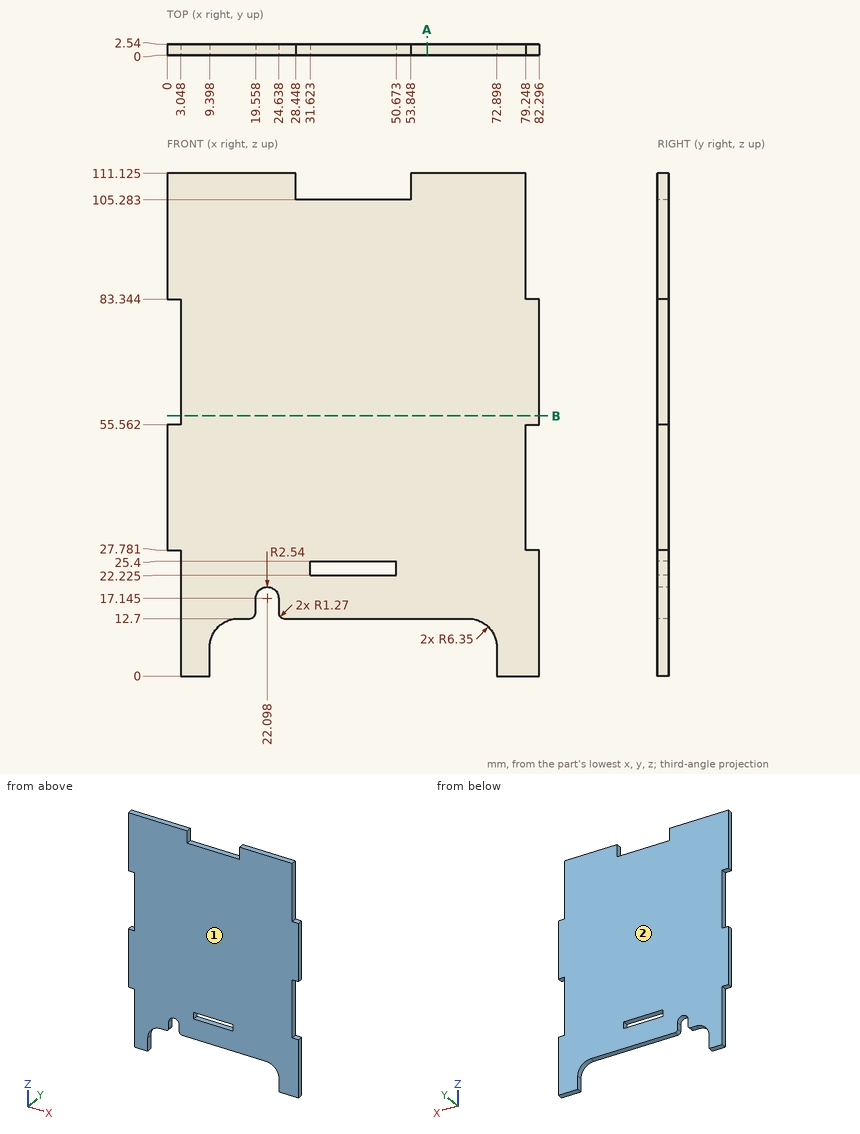
Can you work these out from the drawing? Everything is in mm from the part's minimum corner. Coordinates: 2 decimals unless noted, no trailing zeros. Loops run counter-clockwise (first coordinate to the right, second up) from the corner with the lowest first, then second, coordinate; pieces in that order, holes last. Notation, with made-up numbers: (71.25, -19) -> (82.25, -19) arc R24 ccw to (82.25, -9) -> close; hole circle Ø10 at (9.25, -29.75). An arc over 180 degrees is marked (long way). Return JSON: item names as keys, results as strings.
1) If we section it at A-A, the plane x = 57.5: Write out the boundary of the cut face in (y, z) (1 decimal), then the cut area to 3 significant figures.
Results below:
{"outline": "(0, 12.7) -> (2.5, 12.7) -> (2.5, 111.1) -> (0, 111.1) -> close", "area": "250 mm²"}
2) Thinking about a two-plate mould opening in Y: for the marked faces 1 and 2, which applies, +Y half, -Y half, draft (parallel to the pull), parting line (faces both ways), or undercut?
Results below:
{"face 1": "-Y half", "face 2": "+Y half"}
3) I need wall thicknesses on line 1 (Z direction, x = 50, y = 1.25) (1 decimal); line 2 (Z direction, x = 65, y = 1.5) (1 decimal); line 3 (X direction, y = 0.75, z = 89). Which ranges of each line are inside material? Lowest first, please. Write a range as from..to.
Results below:
{"line 1": "12.7..22.2, 25.4..105.3", "line 2": "12.7..111.1", "line 3": "0..79.25"}
4) Will these pins go through, and if not, where does the flat tip stop? pin 1 (0.8 mm diameter, centred on x = 81, y = 1, fed in from +Z); pin 2 (0.8 mm diameter, centred on y = 2, z = 3.5, fed in from -X); pin 3 (1.3 mm diameter, centred on x = 42.5, y = 1, fed in from +Z).
Results below:
{"pin 1": "z = 83.34", "pin 2": "x = 3.05", "pin 3": "z = 105.28"}
5) If we section it at B-B, the plane z = 57.5: Write out the boundary of the cut face in (x, y) (1 decimal).
Results below:
{"outline": "(3, 0) -> (82.3, 0) -> (82.3, 2.5) -> (3, 2.5) -> close"}
